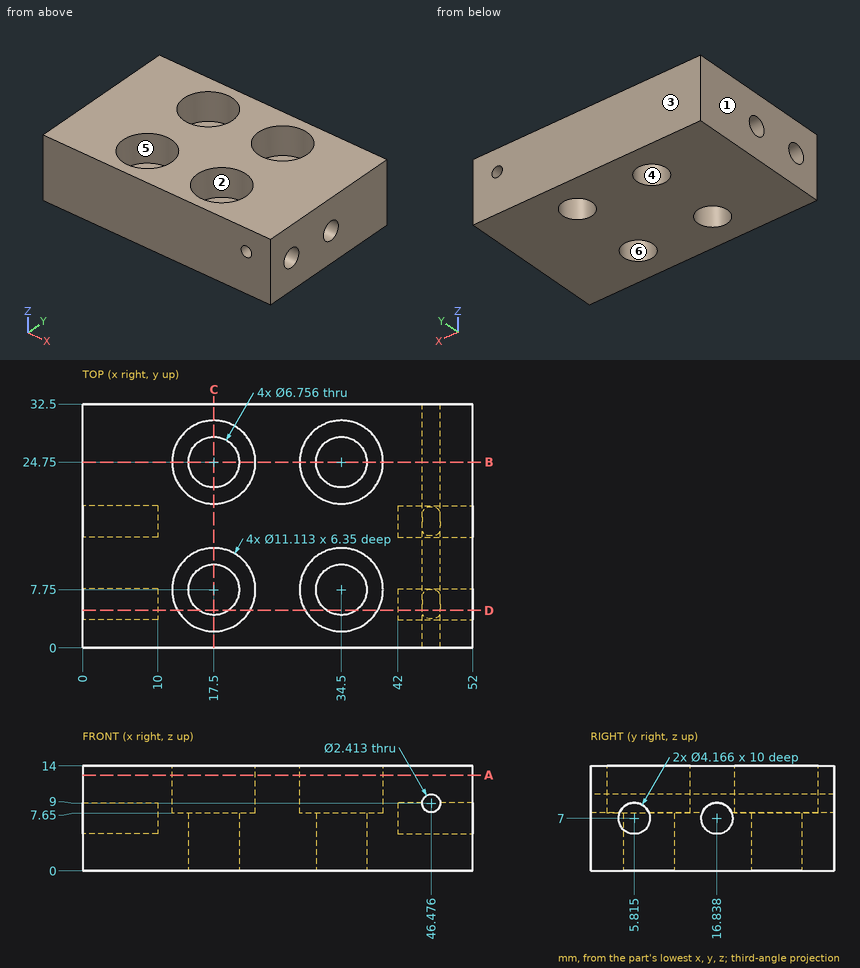
Can you work these out from the drawing? Everything is in mm from the part's minimum corner. A direction names the side the tool comes from. Give positions to 0.01 mm unless a question says otherwise; leave off trailing zeros. Write each loop counter-clockwise with the first axis right and the second up, starting at its lowest first coordinate (ties: lowest second). Pieces come first, ordered by that corner, then holes. Notation, with made-up numbers: (45, -25) -> (93, -25) arc R25 ccw to (93, -12) -> close; hole circle Ø2 at (66, 56.25). An arc over 180 degrees is marked (long way). Write each question's results on one line, items separated by ' | '. Start each with the question number.
Q1. I'm going to push flat-ended pins straight in: pin 1 Ø3.5 at (y, z) = (5, 7) entering from +X; pin 2 Ø9 at (x, y) = (34.5, 7.75) entering from +Z; pin 3 Ø1.2 at (y, z) = (17, 7.5) entering from -X; pin 4 Ø2.5 at (y, z) = (16.84, 7) entering from +X. Where does each tip first touch, or does it pass through?
Q2. Suppose I cut it at C-C, the plane x = 17.5. List the corners of the cut face in (y, z) for me.
Q3. We'd pull the mould along X, two halves only. Please class the marked faces 1, 2, 3 and 4: +X half, -X half, draft (parallel to the pull), parting line (faces both ways), or undercut.
Q4. Suppose I cut it at A-A, the plane z = 12.75. List the corners of the cut face in (x, y) for me, and give its area (3 significant figures).
Q5. Which directions (+Z, -Z, +X, -X, +Y, -Y) give clear straight access to the entire face, cutting with the end or side of a thin tool? Please do the marked faces 5 and 6.
Q6. Suppose I cut it at D-D, the plane y = 5. State how many separate pieces and enclosed holes the cut face has, and give its area (3 significant figures).
Q7. I need wall thicknesses on probe 1 along Y at (x, z) = (49, 7) (1 decimal); probe 2 along Y at (x, z) = (34.5, 12.75); probe 3 along X at (y, z) = (25, 12.5). Which ranges of each line are inside material? Lowest first, please.
Q8. Suppose I cut it at B-B, the plane y = 24.75. List the corners of the cut face in (x, z) for me, and give its area (3 significant figures).
Outcome:
1) pin 1: x = 52 | pin 2: z = 7.65 | pin 3: x = 10 | pin 4: x = 42
2) outline: (0, 0) -> (4.37, 0) -> (4.37, 7.65) -> (2.19, 7.65) -> (2.19, 14) -> (0, 14) -> close; (11.13, 0) -> (21.37, 0) -> (21.37, 7.65) -> (19.19, 7.65) -> (19.19, 14) -> (13.31, 14) -> (13.31, 7.65) -> (11.13, 7.65) -> close; (28.13, 0) -> (32.5, 0) -> (32.5, 14) -> (30.31, 14) -> (30.31, 7.65) -> (28.13, 7.65) -> close
3) face 1: -X half | face 2: undercut | face 3: draft | face 4: undercut
4) outline: (0, 0) -> (52, 0) -> (52, 32.5) -> (0, 32.5) -> close; hole circle Ø11.11 at (17.5, 7.75); hole circle Ø11.11 at (17.5, 24.75); hole circle Ø11.11 at (34.5, 7.75); hole circle Ø11.11 at (34.5, 24.75) | area: 1,300 mm2
5) face 5: +Z | face 6: +Z, -Z
6) separate pieces: 3 | enclosed holes: 0 | area: 466 mm2
7) probe 1: 0 to 3.7, 7.9 to 14.8, 18.9 to 32.5 | probe 2: 0 to 2.19, 13.31 to 19.19, 30.31 to 32.5 | probe 3: 0 to 11.95, 23.05 to 28.95, 40.05 to 52
8) outline: (0, 0) -> (14.12, 0) -> (14.12, 7.65) -> (11.94, 7.65) -> (11.94, 14) -> (0, 14) -> close; (20.88, 0) -> (31.12, 0) -> (31.12, 7.65) -> (28.94, 7.65) -> (28.94, 14) -> (23.06, 14) -> (23.06, 7.65) -> (20.88, 7.65) -> close; (37.88, 0) -> (52, 0) -> (52, 14) -> (40.06, 14) -> (40.06, 7.65) -> (37.88, 7.65) -> close; hole circle Ø2.41 at (46.48, 9) | area: 479 mm2
